Can you work these out from the model? Positions are in its coordinate system, mm. A direction names the side the tool comes from. Give positions to 0.01 mm unless a question says otherwise; leave off trailing zeros. Loops run counter-clockwise (first coordinate to the right, second up) from the corner with the lowest first, then second, coordinate; pieces in that order, holes last. Notation, with made-up numbers: (-9, 55) - (4, 55) arc R19 ccw to (4, 68) - close; hole circle Ø4 at (-35.75, 72). An arc over 180 degrees is marked (long way). Write item = value, one per line.
from build123d import *

# Parameters (mm, degrees)
EXTRUDE_1_DEPTH   = 2
CHAMFER_1_SIZE    = 2
HOLE_WIZARD_M51_D = 5.5


with BuildPart() as part:
    # Эскиз1 → Бобышка-Вытянуть1 (new body)
    with BuildSketch(Plane(origin=(0, 0, 0), x_dir=(1, 0, 0), z_dir=(0, 0, -1))):
        Polygon((10, 0), (-10, 0), (-10, -40), (-20, -40), (-20, -60), (20, -60), (20, -40), (10, -40), align=None)
    extrude(amount=EXTRUDE_1_DEPTH)

    # Фаска1
    chamfer_1_edges = [part.edges().sort_by_distance(p)[0] for p in [
        (-10, 0, -1),
        (10, 0, -1),
        (20, 40, -1),
        (20, 60, -1),
        (-20, 60, -1),
        (-20, 40, -1),
    ]]
    chamfer(chamfer_1_edges, length=CHAMFER_1_SIZE)

    # Отверстие с зазором M51 (through all)
    with Locations(Plane.XY):
        with Locations((-10, 50), (10, 50), (0, 30), (0, 10)):
            Hole(HOLE_WIZARD_M51_D / 2)


solid = part.part
Q1. I need wall thicknesses on L1, parallel to Y at x = 0, z = -1; L2, parallel to X at y = 34.5, z = -0.3; L3, parallel to Y at x = -17.5, z = -1.9. Which ranges of each line are inside material? Lowest first, please.
Output:
L1 = 0 to 7.25, 12.75 to 27.25, 32.75 to 60
L2 = -10 to 10
L3 = 40 to 60
Q2. Which directions (+Z, -Z, +X, -X, +Y, -Y) give clear straight access to the entire face, cutting with the end or side of a thin tool? Please do faces 1 (the flat face through (14, 40, -1)), 2 (the flat face through (-10, 21, -1)), 3 (the flat face through (0, 0, -1)).
Output:
face_1 = +Z, -Z, +X, -Y
face_2 = +Z, -Z, -X, -Y
face_3 = +Z, -Z, +X, -X, -Y
Q3. For pin 1 (1 mm diameter, centred on y = 29, z = -0.5, fed in from +X), with a flat end and sliding along its axis, tell me the tip position at first contact or that it passes through.
Output:
pin_1 = 10
Q4. Imagine slicing it at A-A, the plane z = -0.9. Write out the boundary of the cut face in (x, y).
Output:
outline = (-20, 42) - (-18, 40) - (-10, 40) - (-10, 2) - (-8, 0) - (8, 0) - (10, 2) - (10, 40) - (18, 40) - (20, 42) - (20, 58) - (18, 60) - (-18, 60) - (-20, 58) - close; hole circle Ø5.5 at (-10, 50); hole circle Ø5.5 at (0, 10); hole circle Ø5.5 at (0, 30); hole circle Ø5.5 at (10, 50)
Q5. We'd pull the mould along X, two halves only. Please class faces 4 (the cylindrical face through (10.358, 52.727, -1.014)), 5 (the flat face through (-19, 59, -1)), 6 (the cylindrical face through (0.358, 12.727, -1.014)), 7 (the flat face through (20, 50, -1)): released by +X, released by -X, zero draft, split by the parting line, or undercut.
Output:
face_4 = undercut
face_5 = released by -X
face_6 = undercut
face_7 = released by +X
Q6. Imagine slicing it at B-B, the plane x = -1.5. Write out the boundary of the cut face in (y, z).
Output:
outline = (0, -2) - (7.7, -2) - (7.7, 0) - (0, 0) - close; (12.3, -2) - (27.7, -2) - (27.7, 0) - (12.3, 0) - close; (32.3, -2) - (60, -2) - (60, 0) - (32.3, 0) - close
Q7. Imagine slicing it at D-D, the plane x = -16.5. Write out the boundary of the cut face in (y, z), then the cut area to 3 significant figures.
Output:
outline = (40, -2) - (60, -2) - (60, 0) - (40, 0) - close
area = 40.0 mm2
Q8. Imagine slicing it at C-C, the plane y = 48. Write out the boundary of the cut face in (x, z), then the cut area to 3 significant figures.
Output:
outline = (-20, -2) - (-11.89, -2) - (-11.89, 0) - (-20, 0) - close; (-8.11, -2) - (8.11, -2) - (8.11, 0) - (-8.11, 0) - close; (11.89, -2) - (20, -2) - (20, 0) - (11.89, 0) - close
area = 64.9 mm2
